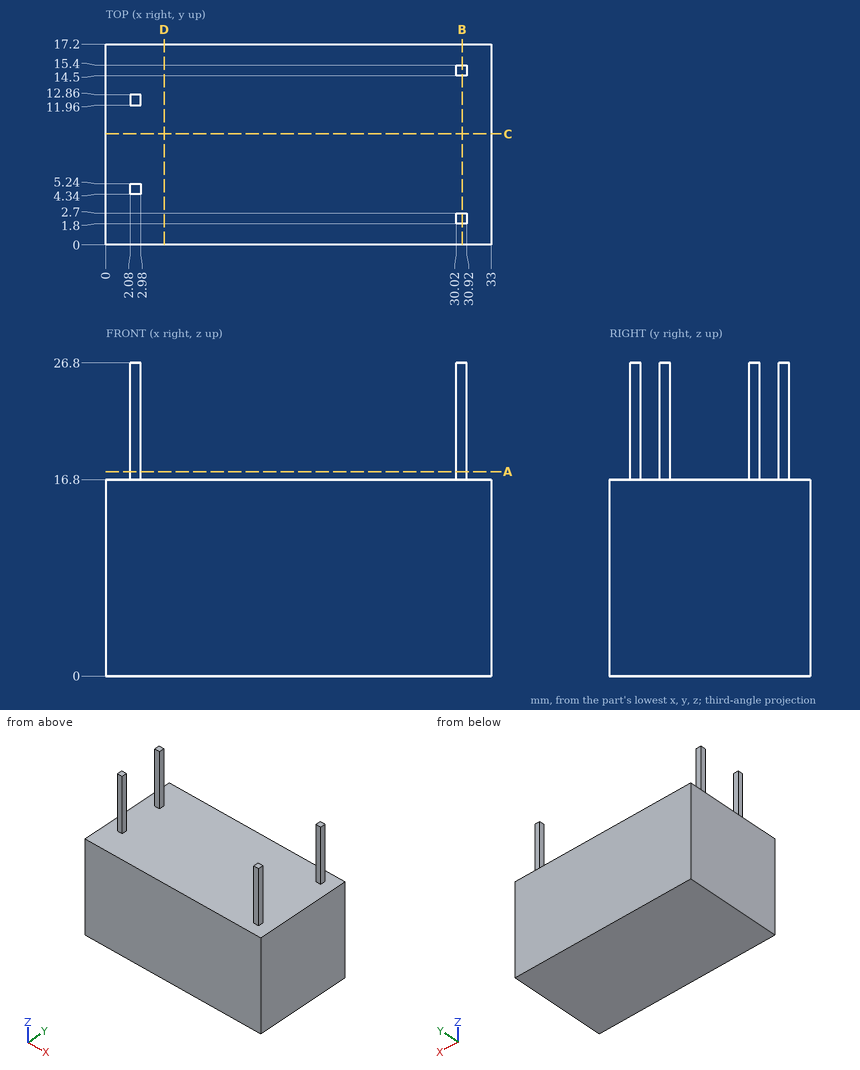
Check sheet for the drawn part. Datum: minimum x, y, z corner. Units: mm. Coordinates: 2 decimals unless noted, no trailing zeros. Order: outer loops, then holes, each group sorted by start corner. A loop starts at its lowest first (then second) coordinate and runs counter-clockwise, first axis right, second up. Notation, with made-up numbers: (-26.75, -37) -> (-16.75, -37) arc R24 ccw to (-16.75, -15) -> close; hole circle Ø9 at (65, 20.25). An arc over 180 degrees is marked (long way). Use a Markdown table: item, result. Add a question column.
1. Cross-section at D-D (x = 5). Enter the section's corners in (y, z).
2. Cross-section at C-C (y = 9.5). Enter the section's corners in (x, z), and give its area (3 significant figures).
3. Material ranges on L1, parallel to Y at x = 30.5, z = 23; L2, parallel to Z at x = 18.5, y = 11; L3, parallel to X at y = 12.5, z = 17, recorded low to high.
4. Go/stop test with flat-tipped pins: pin 1 Ø0.7 at (y, z) = (4.5, 20.5) entering from -X; pin 2 Ø0.7 at (x, z) = (30.5, 22.5) entering from -Y; pin 3 Ø0.7 at (x, z) = (30.5, 21.5) entering from +Y; pin 4 Ø1 at (x, z) = (22.5, 18) entering from +Y. Record where each tip stops, or that it passes through.
5. Cross-section at B-B (x = 30.5). Enter the section's corners in (y, z), and give its area (3 significant figures).
6. Cross-section at A-A (z = 17.5). Enter the section's corners in (x, y).
Filled sheet:
| question | item | result |
|---|---|---|
| 1 | outline | (0, 0) -> (17.2, 0) -> (17.2, 16.8) -> (0, 16.8) -> close |
| 2 | outline | (0, 0) -> (33, 0) -> (33, 16.8) -> (0, 16.8) -> close |
| 2 | area | 554 mm2 |
| 3 | L1 | 1.8 to 2.7, 14.5 to 15.4 |
| 3 | L2 | 0 to 16.8 |
| 3 | L3 | 2.08 to 2.98 |
| 4 | pin 1 | x = 2.08 |
| 4 | pin 2 | y = 1.8 |
| 4 | pin 3 | y = 15.4 |
| 4 | pin 4 | through |
| 5 | outline | (0, 0) -> (17.2, 0) -> (17.2, 16.8) -> (15.4, 16.8) -> (15.4, 26.8) -> (14.5, 26.8) -> (14.5, 16.8) -> (2.7, 16.8) -> (2.7, 26.8) -> (1.8, 26.8) -> (1.8, 16.8) -> (0, 16.8) -> close |
| 5 | area | 307 mm2 |
| 6 | outline | (2.08, 4.34) -> (2.98, 4.34) -> (2.98, 5.24) -> (2.08, 5.24) -> close; (2.08, 11.96) -> (2.98, 11.96) -> (2.98, 12.86) -> (2.08, 12.86) -> close; (30.02, 1.8) -> (30.92, 1.8) -> (30.92, 2.7) -> (30.02, 2.7) -> close; (30.02, 14.5) -> (30.92, 14.5) -> (30.92, 15.4) -> (30.02, 15.4) -> close |
